Design review of the part built by this model. Coordinates are the model's own, in mm. A direction names the side the tool comes from. Round coordinates to 2 decimals unless told otherwise and drop trailing zeros. Order: outer loops, then holes, each group sorted by start corner. A loop starts at its lowest first (then second) coordinate and runs counter-clockwise, first axis right, second up. Notation, with made-up numbers: M 65.25,1 L 76.25,1 A24 cw 76.25,25 Z; hole C 74.25,-38 d6. An arc over 180 degrees is marked long. Write each question's results on one line, items separated by ' | '. Start each with the question number.
Item 1: Take a section at C-C, the plane z = 1. Write out the cut boundary in (x, y), plus the area to 3 significant figures.
Item 2: Take a section at B-B, the plane z = -1. Write out the cut boundary in (x, y).
Item 3: Take a section at A-A, the plane y = 0. Write out the cut boundary in (x, z), plus the area to 3 significant figures.
Item 4: Clearance check with flat-ended pins moving along their axes: pin 1 (3 mm diameter, centred on x = -2, z = -4.5, fed in from -Y); pin 2 (1.5 mm diameter, centred on x = 2.5, y = 1, fed in from -Z). State where each tip first meets the part, or that it passes through.
Item 5: The part is to be moulded in two halves that separate along X. For faces 3 (the cylindrical face through (0, -2, -5)), 4 (the flat face through (-0.74, 1.305, 3.014)), 5 (the flat face through (1, -2, 0)), say which applies: +X half, -X half, draft (parallel to the pull), parting line (faces both ways), or undercut.
Item 6: Machinability: for faces 1 (the flat face through (0, 0, 2)), 2 (the cylindrical face through (-2.579, -1.978, 1.824)), which of the approach directions +Z, -Z, +X, -X, +Y, -Y give a long, thin tool a straight path to every point of the face, cutting with its end or side? Answer none if there is none.
Item 7: Wall thickness on line 1 (Z direction, x = -1.5, y = 2.25); line 2 (X direction, y = -1, z = 2.5); line 3 (X direction, y = 0.25, z = 2.25): over which ranges is each line inside the solid? List them lowest first. Write a range as [from, to].
```python
from build123d import *

# Parameters (mm, degrees)
F2_R      = 2
F3_DEPTH  = 10
F2_R_2    = 3.25
F3_FACE_R = 2
F4_DEPTH  = 4
F5_SIZE   = 0.3
F7_DEPTH  = 2


with BuildPart() as f3:
    # F2 (on Top) → F3 (new body)
    with BuildSketch(Plane.XY):
        Circle(F2_R)
    extrude(amount=-F3_DEPTH)

    # F2 (on Top) + F3_face (on face) → F4 (join)
    with BuildSketch(Plane.XY):
        Circle(F2_R_2)
        Circle(F2_R, mode=Mode.SUBTRACT)
    with BuildSketch(Plane.XY):
        Circle(F3_FACE_R)
    extrude(amount=F4_DEPTH)

    # F5
    f5_edges = [f3.edges().sort_by_distance(p)[0] for p in [
        (-2, 0, -10),
        (-3.25, 0, 4),
    ]]
    chamfer(f5_edges, length=F5_SIZE)

    # F6 (on face) → F7 (cut)
    with BuildSketch(Plane.XY.offset(4)):
        Polygon((1.5, -0.8660254038), (1.5, 0.8660254038), (0, 1.7320508076), (-1.5, 0.8660254038), (-1.5, -0.8660254038), (0, -1.7320508076), align=None)
    extrude(amount=-F7_DEPTH, mode=Mode.SUBTRACT)


solid = f3.part
```
Results list:
1) outline: C 0,0 d6.5 | area: 33.2 mm²
2) outline: C 0,0 d4
3) outline: M -3.25,0 L -2,0 L -2,-9.7 L -1.7,-10 L 1.7,-10 L 2,-9.7 L 2,0 L 3.25,0 L 3.25,3.7 L 2.95,4 L 1.5,4 L 1.5,2 L -1.5,2 L -1.5,4 L -2.95,4 L -3.25,3.7 Z | area: 59.8 mm²
4) pin 1: y = -1.94 | pin 2: z = -9.76
5) face 3: parting line | face 4: undercut | face 5: draft
6) face 1: +Z | face 2: +Z, -Z
7) line 1: [0, 4] | line 2: [-3.09, -1.27], [1.27, 3.09] | line 3: [-3.24, -1.5], [1.5, 3.24]
